Autodesk Inventor part; units mm, degrees
ref_plane "YZ Plane" through (0, 0, 0) normal (1, 0, 0) x (0, 1, 0)
ref_plane "XZ Plane" through (0, 0, 0) normal (0, 1, 0) x (-1, 0, 0)
ref_plane "XY Plane" through (0, 0, 0) normal (0, 0, 1) x (1, 0, 0)
sketch "Sketch1" plane through (0, 0, 0) normal (1, 0, 0) x (0, 1, 0)
  line L0 (0, 0) -> (0, -20)
  line L1 (0, 0) -> (20, 0) construction
  arc A0 (-50, 29.5654) -> (0, -20) centre (3.0398, 33.0683) ccw
  arc A1 (-40.1726, 31.4151) -> (0, 0) centre (8.9221, 52.8024) ccw
  arc A2 (-40.1726, 31.4151) -> (-50.0004, 36.5654) centre (-48.2889, 27.8794) ccw
  arc A3 (-50.0004, 36.5654) -> (-50, 29.5654) centre (-56.0624, 33.0651) ccw
  dimension "d0" = 20
  dimension "d1" = 90
  dimension "d2" = 50
  dimension "d3" = 10
  dimension "d5" = 7
  dimension "d6" = 7
extrude "Extrusion1" add sketch "Sketch1" along normal blind 3.5
properties part number "leg"
Here's how the part is built. I have some questions about the finished solid (model axes, mm). Round coordinates to 2 decimals unless told otherwise and drop trailing zeros. Loops run counter-clockwise (first coordinate to the right, second up) from the corner with the lowest first, then second, coordinate; pieces in that order, holes last. Notation, with made-up numbers: (7, 34) -> (42, 34) arc R19 cw to (42, 53) -> close; hole circle Ø3 at (74.25, 45). An arc over 180 degrees is marked (long way). Answer as CSV lines item,"result".
1. If I drill on L1, parallel to Y at x = 1.65, z = -3; L2, parallel to Y at x = 2.6, z = 33; L3, parallel to Z at x = 0.6, y = -45.5, over which ranges is the centre line in solid material (lowest first)?
Final values:
L1,"y = -36.01 to 0"
L2,"y = -63.06 to -41.07"
L3,"z = 11.4 to 36.28"
2. If we section it at B-B on y = -48.5: Please give me the cut outline in (x, z), plus the area to 3 significant figures.
Final values:
outline,"(0, 20.06) -> (3.5, 20.06) -> (3.5, 36.73) -> (0, 36.73) -> close"
area,"58.3 mm^2"
3. If we section it at A-A on x = 0.7: Please give me the cut outline in (y, z).
Final values:
outline,"(-50, 29.57) arc R53.16 ccw to (0, -20) -> (0, 0) arc R53.55 cw to (-40.17, 31.42) arc R8.85 ccw to (-50, 36.57) arc R7 ccw (long way) to start"
4. For pin 1 (2 mm diameter, centred on x = 0.5, y = -38, fed in from -Z); pin 2 (1 mm diameter, centred on x = 1.5, y = -43, fed in from +Z); pin 3 (10 mm diameter, centred on y = -54, z = 19.5, fed in from +X); pin 4 (1 mm diameter, centred on x = 1.5, y = -56, fed in from -Z), each with a flat end and sliding along its axis, tell me the tip position at first contact or that it passes through.
Final values:
pin 1,"stops at z = -1.89"
pin 2,"stops at z = 35.33"
pin 3,"passes through"
pin 4,"stops at z = 26.07"
5. Thinking about a two-plate mould opening in Y: for faces 1 (the face through (1.726, -63.058, 32.808)), 2 (the face through (2, 0, -10)), 3 (the face through (3.5, -29, 8)), which applies, released by +Y, released by -Y, zero draft, split by the parting line, or undercut?
Final values:
face 1,"undercut"
face 2,"released by +Y"
face 3,"zero draft"
6. If we section it at C-C on z = 33.5: Please give me the cut outline in (x, y), plus the area to 3 significant figures.
Final values:
outline,"(0, -63.05) -> (3.5, -63.05) -> (3.5, -41.45) -> (0, -41.45) -> close"
area,"75.6 mm^2"
